```python
from build123d import *

# Parameters (mm, degrees)
F0_W     = 20
F0_H     = 20
F1_DEPTH = 20
F3_D     = 5
F4_R     = 3
F6_D     = 5


with BuildPart() as f1:
    # F0 (on Top) → F1 (new body)
    with BuildSketch(Plane.XY):
        with Locations((10, -10)):
            Rectangle(F0_W, F0_H)
    extrude(amount=F1_DEPTH)

    # F3 (through all)
    with Locations(Plane.XY.offset(20)):
        with Locations((10, -10)):
            Hole(F3_D / 2)

    # F4
    f4_edges = [f1.edges().sort_by_distance(p)[0] for p in [
        (10, -20, 20),
        (0, -10, 20),
        (20, -10, 20),
        (10, 0, 20),
        (0, -20, 10),
        (20, -20, 10),
        (20, 0, 10),
        (0, 0, 10),
        (10, 0, 0),
        (0, -10, 0),
        (10, -20, 0),
        (20, -10, 0),
    ]]
    fillet(f4_edges, radius=F4_R)

    # F6 (through all)
    with Locations(Plane(origin=(0, 0, 0), x_dir=(0, -1, 0), z_dir=(-1, 0, 0))):
        with Locations((10, 10)):
            Hole(F6_D / 2)


solid = f1.part
```
Check sheet for the modelled part. Datum: model origin and axes. Units: mm. Give positions to 0.01 mm unless a question says otherwise; leave off trailing zeros. Order: outer loops, then holes, each group sorted by start corner. A loop starts at its lowest first (then second) coordinate and runs counter-clockwise, first axis right, second up. Notation, with made-up numbers: (-21, 73) -> (26, 73) arc R22 ccw to (26, 109) -> close; hole circle Ø8 at (13.5, 76.25). An arc over 180 degrees is marked (long way). Use CSV: the item, a comma, the result in double quotes. Start each with the question number.
1) Sectioned sample at C-C, the plane z = 6.5. Record the boundary of the cut face in (x, y).
2) Sectioned sample at A-A, the plane y = -10. Record the boundary of the cut face in (x, z).
3) Material ranges on line 1 (Y direction, x = 10, z = 17); line 2 (Z direction, x = 7, y = -10); line 3 (Y direction, x = 11, z = 16), recorded low to high. Write a range as from..to.
4) Sectioned sample at B-B, the plane x = 11.5. Record the boundary of the cut face in (y, z), plus the area to 3 significant figures.
5) Sectioned sample at D-D, the plane x = 13.5. Record the boundary of the cut face in (y, z).
6) Mould release check, pull along Y, two halves, no side actions. Record for faces 1 (the face through (7.69, -10.96, 3.82)), 2 (the face through (10, -20, 10)), 3 (the face through (0.86, -0.9, 10.1)), 4 (the face through (8.66, -7.89, 16.04)): released by +Y, released by -Y, zero draft, split by the parting line, or undercut.
Recorded:
1,outline,"(0, -17) arc R3 ccw to (3, -20) -> (17, -20) arc R3 ccw to (20, -17) -> (20, -3) arc R3 ccw to (17, 0) -> (3, 0) arc R3 ccw to (0, -3) -> close; hole circle Ø5 at (10, -10)"
2,outline,"(0, 3) arc R3 ccw to (3, 0) -> (7.5, 0) -> (7.5, 7.5) -> (0, 7.5) -> close; (0, 12.5) -> (7.5, 12.5) -> (7.5, 20) -> (3, 20) arc R3 ccw to (0, 17) -> close; (12.5, 0) -> (17, 0) arc R3 ccw to (20, 3) -> (20, 7.5) -> (12.5, 7.5) -> close; (12.5, 12.5) -> (20, 12.5) -> (20, 17) arc R3 ccw to (17, 20) -> (12.5, 20) -> close"
3,line 1,"-20..-12.5, -7.5..0"
3,line 2,"0..7.5, 12.5..20"
3,line 3,"-20..-12.29, -7.71..0"
4,outline,"(-20, 3) arc R3 ccw to (-17, 0) -> (-12, 0) -> (-12, 8.5) arc R2.5 cw to (-12, 11.5) -> (-12, 20) -> (-17, 20) arc R3 ccw to (-20, 17) -> close; (-8, 0) -> (-3, 0) arc R3 ccw to (0, 3) -> (0, 17) arc R3 ccw to (-3, 20) -> (-8, 20) -> (-8, 11.5) arc R2.5 cw to (-8, 8.5) -> close"
4,area,"310 mm2"
5,outline,"(-20, 3) arc R3 ccw to (-17, 0) -> (-3, 0) arc R3 ccw to (0, 3) -> (0, 17) arc R3 ccw to (-3, 20) -> (-17, 20) arc R3 ccw to (-20, 17) -> close; hole circle Ø5 at (-10, 10)"
6,face 1,"undercut"
6,face 2,"released by -Y"
6,face 3,"released by +Y"
6,face 4,"undercut"
